```python
from build123d import *

# Parameters (mm, degrees)
F0_R     = 5.935781
F1_DEPTH = 5.08
F2_R     = 38.1
F3_DEPTH = 50.8
F4_R     = 5.08


with BuildPart() as f1:
    # F0 (on Front) → F1 (new body)
    with BuildSketch(Plane.XZ):
        Circle(F0_R)
    extrude(amount=F1_DEPTH)

    # F2 (on face) → F3 (join)
    with BuildSketch(Plane(origin=(0, 0, 0), x_dir=(-1, 0, 0), z_dir=(0, 1, 0))):
        Circle(F2_R)
    extrude(amount=F3_DEPTH)

    # F4
    f4_edges = [f1.edges().sort_by_distance(p)[0] for p in [
        (38.1, 0, 0),
        (38.1, 50.8, 0),
    ]]
    fillet(f4_edges, radius=F4_R)


solid = f1.part
```
Work out the finished part from the listing and answer in its coordinate system (mm). A direction names the side the tool comes from. Give positions to 0.01 mm unless a question says otherwise; leave off trailing zeros. Order: outer loops, then holes, each group sorted by start corner. A loop starts at its lowest first (then second) coordinate and runs counter-clockwise, first axis right, second up.
1. Section A-A, the plane x = 0 is taken. Determine the outline of the cut face in (y, z), and give its area (3 significant figures).
Result sheet:
outline: (-5.08, -5.94) - (0, -5.94) - (0, -33.02) arc R5.08 ccw to (5.08, -38.1) - (45.72, -38.1) arc R5.08 ccw to (50.8, -33.02) - (50.8, 33.02) arc R5.08 ccw to (45.72, 38.1) - (5.08, 38.1) arc R5.08 ccw to (0, 33.02) - (0, 5.94) - (-5.08, 5.94) - close
area: 3,910 mm2
2. For faces 1 (the cylindrical face through (5.662, -2.504, 1.783)), 2 (the flat face through (0, -5.08, 0)), determine the directions among +Z, -Z, +X, -X, +Y, -Y from which every point of the face is accessible in a straight line to the end or side of a thin tool.
Result sheet:
face 1: -Y
face 2: +Z, -Z, +X, -X, -Y
3. Each of these flat-tipped pins is pushed along its axis until it touches: P1, Ø4, axis at x = 20.5, y = 41.5, coming from the +Z side; P2, Ø6, axis at y = 17, z = -5.5, coming from the -X side; P3, Ø20, axis at x = -2.5, z = -9.5, coming from the -Y side; P4, Ø12, axis at x = 26, y = 19, coming from the -Z side. Where does it stop, or does it pass through?
Result sheet:
P1: stops at z = 33.31
P2: stops at x = -38.02
P3: stops at y = -5.08
P4: stops at z = -32.43
4. Section B-B, the plane z = 0 is taken. Determine the outline of the cut face in (x, y).
Result sheet:
outline: (-38.1, 5.08) arc R5.08 ccw to (-33.02, 0) - (-5.94, 0) - (-5.94, -5.08) - (5.94, -5.08) - (5.94, 0) - (33.02, 0) arc R5.08 ccw to (38.1, 5.08) - (38.1, 45.72) arc R5.08 ccw to (33.02, 50.8) - (-33.02, 50.8) arc R5.08 ccw to (-38.1, 45.72) - close
5. Section C-C, the plane y = 30.5 is taken. Determine the outline of the cut face in (x, z).
Result sheet:
outline: circle Ø76.2 at (0, 0)
6. Straight lines are drawn through the part: L1, parallel to Y at x = -21.5, z = -22; L2, parallel to X at y = 9.5, z = 19; L3, parallel to Z at x = -11.5, y = 31. For each, find the intervals that lie inside material, in ascending order.
Result sheet:
L1: y = 0 to 50.8
L2: x = -33.02 to 33.02
L3: z = -36.32 to 36.32
